Study the drawing (mm; zero at the part's minimum x, y, z) and answer. A direction names the side the tool comes from. Coordinates: 2 decimals unless noted, no trailing zeros. Order: outer loops, then holes, each group sorted by start corner. A loop starts at its lowest first (then second) coordinate and runs counter-clockwise, first axis right, second up. Notation, with made-up numbers: (-26.5, 24) -> (-0.5, 24) arc R14 ccw to (-0.5, 41) -> close; hole circle Ø1 at (63, 2.25). An arc over 180 degrees is marked (long way). Write each question's results on one line, items separated by ' | '. Start each with the question number.
(1) The part is cut by section B-B, the plane z = 12.75. Give the vertices of the cut face in (x, y), then the cut area to 3 significant figures.
(2) The part is cut by section D-D, the plane y = 1.5. Give the vertices of the cut face in (x, z), then the cut area to 3 significant figures.
(3) The part is cut by section A-A, the plane y = 3.75. Give the vertices of the cut face in (x, z).
(4) A tool of negligible diameter and unlimited length cuts with its end or side. For the marked faces 1 and 2, from which of +Z, -Z, +X, -X, +Y, -Y can it reach the whole face along a straight path? Write none if from no direction.
(5) Straight lines are drawn through the part: L1, parallel to X at y = 5.75, z = 17.25; L2, parallel to Z at x = 11.25, y = 4.5. For each, find the intervals that lie inside material, in ascending order.
(6) The part is cut by section C-C, the plane z = 3.5. Give the vertices of the cut face in (x, y) (1 decimal).
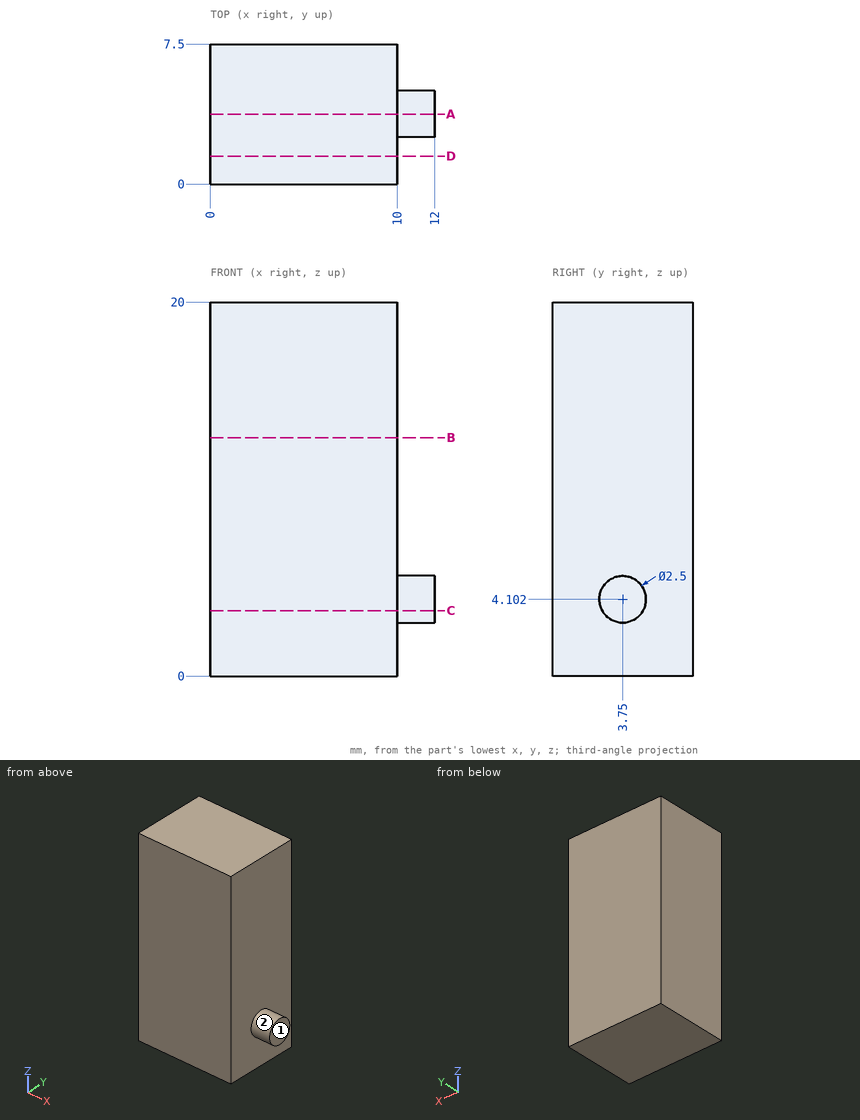
Established:
1) outline: (0, 0) -> (10, 0) -> (10, 7.5) -> (0, 7.5) -> close | area: 75.0 mm^2
2) outline: (0, 0) -> (10, 0) -> (10, 20) -> (0, 20) -> close | area: 200 mm^2
3) outline: (0, 0) -> (10, 0) -> (10, 2.85) -> (12, 2.85) -> (12, 5.35) -> (10, 5.35) -> (10, 20) -> (0, 20) -> close
4) face 1: +Z, -Z, +X, +Y, -Y | face 2: +X
5) L1: x = 0 to 10 | L2: z = 3.1 to 5.1
6) outline: (0, 0) -> (10, 0) -> (10, 2.7) -> (12, 2.7) -> (12, 4.8) -> (10, 4.8) -> (10, 7.5) -> (0, 7.5) -> close
